Autodesk Inventor part; units mm, degrees
ref_plane "Work Plane1" through (0, 0, -15) normal (0, 0, 1) x (1, 0, 0)
ref_plane "YZ Plane" through (0, 0, 0) normal (1, 0, 0) x (0, 1, 0)
ref_plane "XZ Plane" through (0, 0, 0) normal (0, 1, 0) x (-1, 0, 0)
sketch "Sketch1" plane through (0, 0, 0) normal (0, 0, 1) x (1, 0, 0)
  line L0 (0, 0) -> (25, 0)
  line L1 (25, 0) -> (25, 40)
  line L2 (25, 40) -> (0, 40)
  line L3 (0, 40) -> (0, 0)
  dimension "d1" = 25
  dimension "d2" = 40
  dimension "d3" = 25
extrude "Extrusion1" add sketch "Sketch1" against normal blind 30
sketch "Sketch2" plane through (25, 0, 0) normal (1, 0, 0) x (0, 0, -1)
  line L0 (0, 0) -> (30, 0)
  circle A0 centre (15, 6.56) radius 2.46
extrude "Extrusion2" cut sketch "Sketch2" against normal blind 30
sketch "Sketch3" plane through (0, 0, 0) normal (-1, 0, 0) x (0, 0, 1)
  line L0 (0, 0) -> (-30, 0)
  line L1 (-25.05, 0) -> (-4.95, 0)
  line L2 (-4.95, 0) -> (-4.95, 33.12)
  line L3 (-4.95, 33.12) -> (-25.05, 33.12)
  line L4 (-25.05, 33.12) -> (-25.05, 0)
  dimension "d11" = 20.1
extrude "Extrusion3" cut sketch "Sketch3" against normal blind 20
sketch "Sketch4" plane through (0, 0, 0) normal (0, -1, 0) x (1, 0, 0)
  line L0 (20, -4.95) -> (20, -25.05)
  line L1 (20, -15) -> (25, -15)
  line L2 (25, 0) -> (25, -30)
  line L3 (20, -8.025) -> (25, -8.025)
  line L4 (25, -8.025) -> (25, -21.975)
  line L5 (25, -21.975) -> (20, -21.975)
  line L6 (20, -21.975) -> (20, -8.025)
  line L7 (20, -8.025) -> (25, -21.975) construction
  line L8 (25, -8.025) -> (20, -21.975) construction
  line L9 (25, -12.54) -> (25, -17.46)
  point P0 (0, 0)
  point P1 (22.5, -15)
  dimension "d14" = 13.95
extrude "Extrusion4" add sketch "Sketch4" along normal blind 15
sketch "Sketch5" plane through (20, 0, 0) normal (-1, 0, 0) x (0, 0, 1)
  circle A0 centre (-15, 6.56) radius 2.46
  circle A1 centre (-15, 6.56) radius 4.7025
  circle A2 centre (-15, 6.56) radius 2.46
  circle A3 centre (-15, 6.56) radius 2.46
  point P0 (0, 0)
  dimension "d17" = 9.405
extrude "Extrusion5" cut sketch "Sketch5" against normal blind 2.1
sketch "Sketch6" plane through (25, 0, 0) normal (1, 0, 0) x (0, 0, -1)
  circle A0 centre (15, 6.56) radius 4.7025
  line L0 (15, 6.56) -> (15, 23.56)
  circle A1 centre (15, 23.56) radius 2.46
  point P0 (0, 0)
  dimension "d20" = 17
  dimension "d21" = 4.92
extrude "Extrusion6" cut sketch "Sketch6" against normal blind 10 contours A1
sketch "Sketch7" plane through (20, 0, 0) normal (-1, 0, 0) x (0, 0, 1)
  circle A0 centre (-15, 23.56) radius 2.46
  circle A1 centre (-15, 23.56) radius 4.7025
  point P0 (0, 0)
  dimension "d24" = 9.405
extrude "Extrusion7" cut sketch "Sketch7" against normal blind 2.1
sketch "Sketch9" plane through (25, 0, 0) normal (1, 0, 0) x (0, 0, -1)
  circle A0 centre (15, 6.56) radius 2.46
  circle A1 centre (15, 6.56) radius 2.46
  circle A2 centre (15, 23.56) radius 2.46
  circle A3 centre (15, 23.56) radius 2.46
  line L0 (30, 40) -> (30, 0)
  line L1 (30, 0) -> (30, 40)
  line L2 (30, 40) -> (0, 40)
  line L3 (0, 40) -> (0, 0)
  line L4 (0, 0) -> (8.025, 0)
  line L5 (21.975, 0) -> (21.975, -15)
  line L6 (21.975, -15) -> (8.025, -15)
  line L7 (8.025, -15) -> (8.025, 0)
  line L8 (0, 0) -> (8.025, 0)
  line L9 (21.975, 0) -> (30, 0)
extrude "Extrusion8" add sketch "Sketch9" along normal blind 5
sketch "Sketch10" plane through (0, 40, 0) normal (0, 1, 0) x (1, 0, 0)
  line L0 (0, 30) -> (30, 30)
  line L1 (30, 0) -> (0, 0)
  line L2 (0, 30) -> (30, 30)
  line L3 (30, 30) -> (30, 0)
  line L4 (30, 0) -> (0, 0)
  line L5 (0, 0) -> (0, 30)
extrude "Extrusion9" add sketch "Sketch10" along normal blind 30
sketch "Sketch12" plane through (30, 0, 0) normal (1, 0, 0) x (0, 0, -1)
  circle A0 centre (15, 6.56) radius 2.46
  line L0 (15, 6.56) -> (15, 15.06)
  circle A1 centre (15, 15.06) radius 2.525
  point P0 (0, 0)
  dimension "d31" = 8.5
  dimension "d33" = 5.05
extrude "Extrusion10" cut sketch "Sketch12" against normal blind 30 contours A1
sketch "Sketch14" plane through (0, 0, 0) normal (0, 0, 1) x (1, 0, 0)
  line L0 (30, 70) -> (0, 70)
  line L1 (0, 100) -> (-8, 100)
  line L2 (30, 0) -> (30, 70)
  line L3 (30, 118) -> (30, 70)
  line L4 (30, 105) -> (30, 100)
  line L5 (0, 70) -> (30, 70)
  line L6 (0, 70) -> (0, 100)
  line L7 (15, 136) -> (30, 118)
  line L8 (-8, 136) -> (15, 136)
  line L9 (-8, 100) -> (-8, 136)
  point P0 (0, 0)
  dimension "d47" = 30
extrude "Extrusion12" add sketch "Sketch14" against normal blind 30
sketch "Sketch15" plane through (0, 0, -25.05) normal (-1, 0, 0) x (0, 0, 1)
  line L0 (0, 33.12) -> (20.1, 33.12)
  line L1 (20.1, 33.12) -> (20.1, 0)
  line L2 (0, 33.12) -> (20.1, 33.12)
  line L3 (20.1, 33.12) -> (20.1, 31.1)
  line L4 (20.1, 31.1) -> (0, 31.1)
  line L5 (0, 31.1) -> (0, 33.12)
  point P0 (25.05, 0)
  dimension "d57" = 2.02
extrude "Extrusion13" add sketch "Sketch15" against normal blind 20
sketch "Sketch23" plane through (0, 0, 0) normal (0, 0, 1) x (1, 0, 0)
  line L0 (0, 100) -> (-8, 100)
  line L1 (-8, 136) -> (15, 136)
  line L2 (-8, 136) -> (15, 136)
  line L3 (30, 118) -> (15, 136)
  line L4 (15, 136) -> (30, 118)
  line L5 (30, 118) -> (30, 93)
  line L6 (30, 0) -> (30, 118)
  line L7 (30, 93) -> (0, 93)
  line L8 (0, 93) -> (0, 100)
  line L9 (-8, 100) -> (0, 100)
  line L10 (15, 136) -> (-8, 136)
  line L11 (-8, 136) -> (-8, 100)
  point P0 (0, 0)
  point P1 (-2, 102)
  point P2 (4, 118)
  point P3 (-2, 134)
  dimension "d85" = 25
extrude "Extrusion14" add sketch "Sketch23" along normal blind 15
ref_plane "Work Plane1" through (0, 0, -15) normal (0, 0, 1) x (1, 0, 0)
mirror "Mirror1" about plane through (0, 0, -15) normal (0, 0, 1) of "Extrusion14"
sketch "Sketch26" plane through (-8, 136, 15) normal (0, 1, 0) x (1, 0, 0)
  line L0 (0, 60) -> (0, 0)
  line L1 (0, 30) -> (0, 10)
  line L2 (0, 10) -> (5, 10)
  line L3 (5, 10) -> (5, 50)
  line L4 (5, 50) -> (0, 50)
  line L5 (0, 50) -> (0, 30)
  line L6 (0, 50) -> (5, 30)
  line L7 (5, 30) -> (0, 10)
  point P0 (8, 15)
  dimension "d88" = 20
  dimension "d89" = 5
  dimension "d90" = 40
  dimension "d91" = 5
extrude "Extrusion15" cut sketch "Sketch26" against normal through all contours L6 L7 L0
properties part number "32mm_x_60mm"
Read the model definition and answer for the solid it produces. Units are mm, in the model's axes. A direction names the side the tool comes from. Coordinates: 2 decimals unless noted, no trailing zeros. Order: outer loops, then holes, each group sorted by start corner. A loop starts at its lowest first (then second) coordinate and runs counter-clockwise, first axis right, second up. Notation, with made-up numbers: M 26,15 L 70,15 A33 cw 70,53 Z; hole C 46.25,1.5 d7. An arc over 180 degrees is marked long. Put each result on its own line as item: value. Start each with the question number.
Item 1: The mould has two halves that part along Y. Classify faces 1 (the face through (15, 93, -37)), 2 (the face through (4, 136, -15)), 3 (the face through (25.995, 24.502, -17.272)), 4 (the face through (10, 15, -4.95)): +Y half, -Y half, draft (parallel to the pull), parting line (faces both ways), or undercut.
Item 2: Section C-C, the plane x = 12 is taken. Determine the outline of the cut face in (y, z).
Item 3: Given pin 1 Ø6 at (x, z) = (7.5, -13.5) entering from -Y; pin 2 Ø8.5 at (y, z) = (6.56, -15) entering from +X; pin 3 Ø6 at (x, y) = (10.5, 9) entering from +Z; pin 4 Ø4.5 at (x, z) = (12.5, 10) entering from -Y, each flat-ended and moving along its own axis, determine where each tip first touches the part or whether it passes through.
Item 4: For faces 5 (the face through (25, -7, -21.975)), 6 (the face through (15, 0, -3)), 7 (the face through (10, 31.1, -15)), 8 (the face through (-2, 100, -15)), 9 (the face through (-5.535, 118.252, -25.14)), determine the directions among +Z, -Z, +X, -X, +Y, -Y from which every point of the face is accessible in a straight line to the end or side of a thin tool.
Item 5: Consider probe 1 along Z at (x, y) = (27.5, 23.56); probe 2 along Y at (x, z) = (21.35, -15) (1 decimal); probe 3 along Y at (x, z) = (21, -15) (1 decimal). Determine where each line is inside the solid, lowest interval first. Write a range as [from, to].
Item 6: Section B-B, the plane z = -32 is taken. Determine the outline of the cut face in (x, y), plus the area to 3 significant figures.
Item 7: Section D-D, the plane y = 60 is taken. Determine the outline of the cut face in (x, z).
Item 8: Section A-A, the plane y = 15.06 is taken. Determine the outline of the cut face in (x, z) (3 decimals), plus the area to 4 significant figures.
Computed:
1. face 1: -Y half
1. face 2: +Y half
1. face 3: undercut
1. face 4: draft
2. outline: M 0,-30 L 93,-30 L 93,-45 L 136,-45 L 136,15 L 93,15 L 93,0 L 0,0 L 0,-4.95 L 31.1,-4.95 L 31.1,-25.05 L 0,-25.05 Z
3. pin 1: stops at y = 31.1
3. pin 2: stops at x = 30
3. pin 3: stops at z = 0
3. pin 4: stops at y = 93
4. face 5: -Z, +X, -X, -Y
4. face 6: +Z, +X, -X, -Y
4. face 7: -X, -Y
4. face 8: +Z, -Z, -X, -Y
4. face 9: -X, +Y, -Y
5. probe 1: z = [-30, -17.46], [-12.54, 0]
5. probe 2: y = [-15, 1.9], [11.3, 12.5], [17.6, 18.9], [28.3, 128.4]
5. probe 3: y = [-15, 1.9], [11.3, 12.5], [17.6, 18.9], [28.3, 128.8]
6. outline: M -7.25,100 L 0,100 L 0,93 L 30,93 L 30,118 L 15,136 L -7.25,136 Z
6. area: 1,420 mm2
7. outline: M 0,-30 L 30,-30 L 30,0 L 0,0 Z
8. outline: M 0,-30 L 30,-30 L 30,-17.525 L 20,-17.525 L 20,-25.05 L 0,-25.05 Z; M 0,-4.95 L 20,-4.95 L 20,-12.475 L 30,-12.475 L 30,0 L 0,0 Z
8. area: 447.5 mm2
